```python
from build123d import *

# Parameters (mm, degrees)
SKETCH_1_R          = 4
EXTRUDE_1_DEPTH     = 4
SKETCH_2_R          = 2
CUT_EXTRUDE_1_DEPTH = 15
SKETCH_4_W          = 16
SKETCH_4_H          = 44
EXTRUDE_2_DEPTH     = 6
SKETCH_5_W          = 10
SKETCH_5_H          = 10
SKETCH_5_R          = 2
EXTRUDE_3_DEPTH     = 6
SKETCH_6_R          = 1.5
CUT_EXTRUDE_2_DEPTH = 54.749418602


with BuildPart() as part:
    # 草图1 → 凸台-拉伸1 (new, symmetric)
    with BuildSketch(Plane(origin=(0, 0, 0), x_dir=(0, 0, -1), z_dir=(1, 0, 0))):
        with BuildLine():
            Line((5.28471901, 7.285035689), (-15, 22))
            Line((-15, 22), (-35, 22))
            Line((-35, 22), (-35, -0.025536126))
            Line((-35, -0.025536126), (-35, -22))
            Line((-35, -22), (-15, -22))
            Line((-15, -22), (5.28471901, -7.285035689))
            ThreePointArc((5.28471901, -7.285035689), (9, 0), (5.28471901, 7.285035689))
        make_face()
        Circle(SKETCH_1_R, mode=Mode.SUBTRACT)
        with BuildLine():
            Line((-4.746449606, 7.646647379), (-15, 14))
            Line((-15, 14), (-27, 14))
            Line((-27, 14), (-27, -14))
            Line((-27, -14), (-15, -14))
            Line((-15, -14), (-4.746449606, -7.646647379))
            ThreePointArc((-4.746449606, -7.646647379), (-9, 0), (-4.746449606, 7.646647379))
        make_face(mode=Mode.SUBTRACT)
    extrude_1 = extrude(amount=EXTRUDE_1_DEPTH, both=True)

    # 草图2 → 切除-拉伸1 (cut)
    with BuildSketch(Plane.XY.offset(35)):
        with Locations((0, 15)):
            Circle(SKETCH_2_R)
        with Locations(Location((0, -15, 0), (0, 0, 30))):
            Circle(SKETCH_2_R)
    cut_extrude_1 = extrude(amount=-CUT_EXTRUDE_1_DEPTH, mode=Mode.SUBTRACT)

    # 草图4 → 凸台-拉伸2 (add)
    with BuildSketch(Plane.XY.offset(35)):
        with Locations((12, 0)):
            Rectangle(SKETCH_4_W, SKETCH_4_H)
    extrude(amount=-EXTRUDE_2_DEPTH)

    # 镜向1: 凸台-拉伸1, 切除-拉伸1 across plane
    add(extrude_1.mirror(Plane(origin=(12, 0, 0), x_dir=(0, 0, 1), z_dir=(1, 0, 0))))
    add(cut_extrude_1.mirror(Plane(origin=(12, 0, 0), x_dir=(0, 0, 1), z_dir=(1, 0, 0))), mode=Mode.SUBTRACT)

    # 草图5 → 凸台-拉伸3 (add)
    # profile 1 of 4: a face of its own
    with BuildSketch(Plane.XY.offset(35)):
        with Locations((-9, 17)):
            Rectangle(SKETCH_5_W, SKETCH_5_H)
        with Locations((-9, 17)):
            Circle(SKETCH_5_R, mode=Mode.SUBTRACT)
    # profile 2 of 4: a face of its own
    with BuildSketch(Plane.XY.offset(35)):
        with Locations((33, 17)):
            Rectangle(SKETCH_5_W, SKETCH_5_H)
        with Locations(Location((33, 17, 0), (0, 0, 180))):
            Circle(SKETCH_5_R, mode=Mode.SUBTRACT)
    # profile 3 of 4: a face of its own
    with BuildSketch(Plane.XY.offset(35)):
        with Locations((33, -17)):
            Rectangle(SKETCH_5_W, SKETCH_5_H)
        with Locations((33, -17)):
            Circle(SKETCH_5_R, mode=Mode.SUBTRACT)
    # profile 4 of 4: a face of its own
    with BuildSketch(Plane.XY.offset(35)):
        with Locations((-9, -17)):
            Rectangle(SKETCH_5_W, SKETCH_5_H)
        with Locations(Location((-9, -17, 0), (0, 0, 180))):
            Circle(SKETCH_5_R, mode=Mode.SUBTRACT)
    extrude(amount=-EXTRUDE_3_DEPTH)

    # 草图6 → 切除-拉伸2 (cut, through all)
    with BuildSketch(Plane(origin=(0, 0, 4), x_dir=(-1, 0, 0), z_dir=(0, 0, -1))):
        Circle(SKETCH_6_R)
    extrude(amount=CUT_EXTRUDE_2_DEPTH, mode=Mode.SUBTRACT)


solid = part.part
```
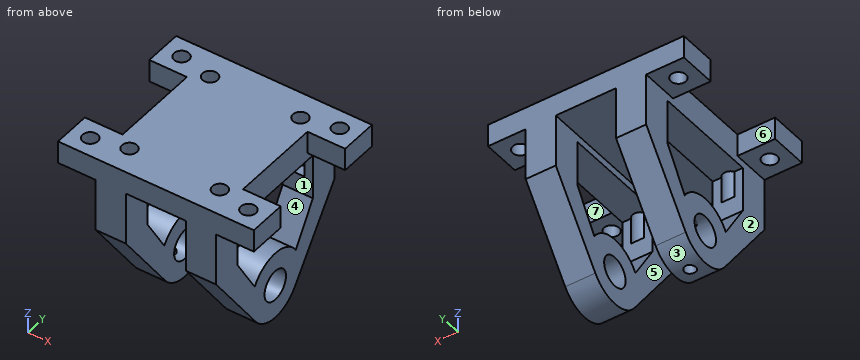
Part model, mm, in its own coordinate system. Face numbers are marked on the shaded views. A direction names the side the tool comes from. Give positions to 0.01 mm unless a question says otherwise; leave off trailing zeros. Write each loop counter-clockwise with the first axis right and the second up, starting at its lowest first coordinate (ties: lowest second). Pieces come first, ordered by that corner, then holes. Notation, with made-up numbers: (75, -14.5) -> (126, -14.5) arc R23 ccw to (126, 23.5) -> close; hole circle Ø6 at (11.25, 42). An arc over 180 degrees is marked (long way). Put each result on its own line as item: value. Start each with the question number.
Item 1: Cut at A-A (x = 24). List the corners of the cut face in (y, z), then the cut area to 3 significant figures.
Item 2: Wall check: L1, parallel to Y at x = 33, z = 31.3; L2, parallel to X at y = -12, z = 3; L3, parallel to X at y = 15, z = 27. Give the ranges that are in metal, low to high. Write a range as [from, to].
Item 3: Which spindle directions (+Z, -Z, +X, -X, +Y, -Y) get a long thin tool onto all of the face, cutting with end or side? Do the marked faces 4, 5, 6 and 7. Say none if no direction does.
Item 4: Cut at D-D (x = 5.5). List the corners of the cut face in (y, z).
Item 5: Cut at B-B (x = 29.5). List the corners of the cut face in (y, z), then the cut area to 3 significant figures.
Item 6: Pin check, flat tips, straight feed: pin 1 Ø6 at (x, z) = (0, 8.5) entering from -Y; pin 2 Ø13 at (y, z) = (8.5, 15.5) entering from -X; pin 3 Ø1.5 at (y, z) = (11, 28) entering from +X; pin 4 Ø6 at (x, y) = (-1.5, -1.5) entering from -Z. Stop position of each tip, or through.
Item 7: Pull direction Z, two halves, no side cores. Call the marked faces 1, 2 and 3: pulls with the +Z half, pulls with the -Z half, needs draft (parallel to the pull), parting line crosses it, or undercut.
Item 8: Cut at C-C (z = 0). List the corners of the cut face in (x, y).
Answer list:
1. outline: (-22, 15) -> (-7.29, -5.28) arc R9 ccw to (7.29, -5.28) -> (22, 15) -> (22, 35) -> (17, 35) -> (17, 20) -> (14, 20) -> (14, 15) -> (7.65, 4.75) arc R9 ccw to (-7.65, 4.75) -> (-14, 15) -> (-14, 20) -> (-17, 20) -> (-17, 35) -> (-22, 35) -> close; (-13, 27) -> (13, 27) -> (13, 35) -> (-13, 35) -> close; hole circle Ø8 at (0, 0)
1. area: 844 mm2
2. L1: y = [-22, -19], [-15, -12], [12, 15], [19, 22]
2. L2: x = [-4, 4], [20, 28]
2. L3: x = [-4, -2], [2, 4], [20, 22], [26, 28]
3. face 4: +X, -X
3. face 5: -Z, +Y, -Y
3. face 6: +Z, -Z, -X
3. face 7: +Z, -Z, +X
4. outline: (-22, 29) -> (22, 29) -> (22, 35) -> (-22, 35) -> close
5. outline: (-22, 29) -> (-12, 29) -> (-12, 35) -> (-22, 35) -> close; (12, 29) -> (22, 29) -> (22, 35) -> (12, 35) -> close
5. area: 120 mm2
6. pin 1: stops at y = -19.46
6. pin 2: stops at x = -4
6. pin 3: stops at x = 28
6. pin 4: stops at z = -9
7. face 1: undercut
7. face 2: needs draft
7. face 3: pulls with the -Z half
8. outline: (-4, -11.12) -> (4, -11.12) -> (4, -4) -> (-4, -4) -> close; (-4, 4) -> (4, 4) -> (4, 11.12) -> (-4, 11.12) -> close; (20, -11.12) -> (28, -11.12) -> (28, -4) -> (20, -4) -> close; (20, 4) -> (28, 4) -> (28, 11.12) -> (20, 11.12) -> close
